Autodesk Inventor part; units mm, degrees
ref_plane "YZ Plane" through (0, 0, 0) normal (1, 0, 0) x (0, 1, 0)
ref_plane "XZ Plane" through (0, 0, 0) normal (0, 1, 0) x (-1, 0, 0)
ref_plane "XY Plane" through (0, 0, 0) normal (0, 0, 1) x (1, 0, 0)
sketch "Sketch1" plane through (0, 0, 0) normal (0, 0, 1) x (1, 0, 0)
  line L0 (-20, -20) -> (20, -20)
  line L1 (20, -20) -> (20, 20)
  line L2 (20, 20) -> (-20, 20)
  line L3 (-20, 20) -> (-20, -20)
  line L4 (-20, -20) -> (20, 20) construction
  line L5 (20, -20) -> (-20, 20) construction
  point P0 (0, 0)
  dimension "d0" = 40
  dimension "d1" = 40
extrude "Extrusion1" add sketch "Sketch1" along normal blind 5
sketch "Sketch2" plane through (0, 0, 5) normal (0, 0, 1) x (1, 0, 0)
  line L0 (-10, -10) -> (10, -10)
  line L1 (10, -10) -> (10, 10)
  line L2 (10, 10) -> (-10, 10)
  line L3 (-10, 10) -> (-10, -10)
  line L4 (-10, -10) -> (10, 10) construction
  line L5 (10, -10) -> (-10, 10) construction
  point P0 (0, 0)
  dimension "d4" = 20
  dimension "d5" = 20
extrude "Extrusion2" add sketch "Sketch2" along normal blind 5
sketch "Sketch3" plane through (0, 0, 0) normal (0, 0, -1) x (-1, 0, 0)
  line L0 (-20, -20) -> (20, -20)
  line L1 (20, -20) -> (20, 20)
  line L2 (20, 20) -> (-20, 20)
  line L3 (-20, 20) -> (-20, -20)
  line L4 (-20, -20) -> (20, 20) construction
  line L5 (20, -20) -> (-20, 20) construction
  line L6 (-10.1, -10) -> (10.1, -10)
  line L7 (10.1, -10) -> (10.1, 20)
  line L8 (10.1, 20) -> (-10.1, 20)
  line L9 (-10.1, 20) -> (-10.1, -10)
  line L10 (-10.1, -10) -> (10.1, 20) construction
  line L11 (10.1, -10) -> (-10.1, 20) construction
  point P0 (0, 0)
  point P1 (0, 5)
  dimension "d8" = 40
  dimension "d9" = 40
  dimension "d10" = 20.2
  dimension "d11" = 30
  dimension "d55" = 20
extrude "Extrusion3" add sketch "Sketch3" along normal blind 40.1 contours L3 L2 L9 L6 L7 L1 L0
sketch "Sketch4" plane through (0, 0, 0) normal (0, 0, -1) x (-1, 0, 0)
  circle A0 centre (0, 0) radius 7.5
  dimension "d14" = 15
extrude "Extrusion4" cut sketch "Sketch4" against normal blind 6
sketch "Sketch6" plane through (20, -20, -40.1) normal (1, 0, 0) x (0, 0, -1)
  line L0 (-45.1, 40) -> (-37.1, 40)
  line L1 (-37.1, 40) -> (-37.1, 0)
  line L2 (-37.1, 0) -> (-45.1, 0)
  line L3 (-45.1, 0) -> (-45.1, 40)
  line L4 (-45.1, 40) -> (-37.1, 0) construction
  line L5 (-37.1, 40) -> (-45.1, 0) construction
  line L6 (0, 40) -> (-45.1, 40)
  line L7 (-45.1, 0) -> (0, 0)
  line L8 (-45.1, 0) -> (-45.1, 40)
  point P0 (-40.1, 20)
  point P1 (-41.1, 20)
  point P2 (-40.1, 40)
  point P3 (-45.1, 50)
  dimension "d19" = 8
extrude "Extrusion6" add sketch "Sketch6" along normal blind 15
mirror "Mirror1" about plane through (0, 0, 0) normal (1, 0, 0) of "Extrusion6"
sketch "Sketch7" plane through (0, 0, 5) normal (0, 0, 1) x (1, 0, 0)
  circle A0 centre (27.5, 10) radius 2.05
  circle A1 centre (27.5, -10) radius 2.05
  circle A2 centre (-27.5, -10) radius 2.05
  circle A3 centre (-27.5, 10) radius 2.05
  line L0 (35, 20) -> (35, -20)
  line L1 (-35, 20) -> (-35, -20)
  line L2 (35, -20) -> (-35, -20)
  line L3 (-35, 20) -> (35, 20)
  line L4 (-20, 20) -> (-35, 20)
  point P0 (0, 0)
  point P1 (20, 20)
  dimension "d22" = 4.1
  dimension "d23" = 4.1
  dimension "d24" = 4.1
  dimension "d25" = 4.1
  dimension "d26" = 7.5
  dimension "d27" = 7.5
  dimension "d28" = 7.5
  dimension "d29" = 7.5
  dimension "d30" = 10
  dimension "d31" = 10
  dimension "d32" = 10
  dimension "d33" = 10
extrude "Extrusion7" cut sketch "Sketch7" against normal through all contours A0 | A1 | A2 | A3
sketch "Sketch9" plane through (20, -20, -3) normal (0, 0, -1) x (-1, 0, 0)
  circle A0 centre (-7.5, 30) radius 2.05
  circle A1 centre (-7.5, 10) radius 2.05
  circle A2 centre (47.5, 30) radius 2.05
  circle A3 centre (47.5, 10) radius 2.05
  circle A4 centre (-7.5, 30) radius 5
  circle A5 centre (-7.5, 10) radius 5
  circle A6 centre (47.5, 30) radius 5
  circle A7 centre (47.5, 10) radius 5
  point P0 (20, 20)
  dimension "d39" = 10
  dimension "d40" = 10
  dimension "d41" = 10
  dimension "d42" = 10
extrude "Extrusion8" cut sketch "Sketch9" against normal blind 5 contours A0 | A1 | A4 | A5 | A6 | A7
sketch "Sketch10" plane through (-20, -20, -40.1) normal (-1, 0, 0) x (0, 0, 1)
  line L0 (22.1, 17.5) -> (37.1, 17.5)
  line L1 (37.1, 17.5) -> (37.1, 32.5)
  line L2 (37.1, 32.5) -> (22.1, 32.5)
  line L3 (22.1, 32.5) -> (22.1, 17.5)
  line L4 (22.1, 17.5) -> (37.1, 32.5) construction
  line L5 (37.1, 17.5) -> (22.1, 32.5) construction
  line L6 (37.1, 0) -> (37.1, 40)
  line L7 (40.1, 10) -> (0, 10)
  point P0 (40.1, 20)
  point P1 (29.6, 25)
  dimension "d45" = 15
  dimension "d46" = 15
  dimension "d47" = 7.5
extrude "Extrusion9" cut sketch "Sketch10" against normal through all
sketch "Sketch11" plane through (-20, -20, -40.1) normal (0, -1, 0) x (1, 0, 0)
  line L0 (27.5, 22.1) -> (12.5, 22.1)
  line L1 (12.5, 22.1) -> (12.5, 37.1)
  line L2 (12.5, 37.1) -> (27.5, 37.1)
  line L3 (27.5, 37.1) -> (27.5, 22.1)
  line L4 (27.5, 22.1) -> (12.5, 37.1) construction
  line L5 (12.5, 22.1) -> (27.5, 37.1) construction
  line L6 (0, 37.1) -> (-15, 37.1)
  line L7 (0, 0) -> (0, 37.1)
  point P0 (20, 40.1)
  point P1 (20, 29.6)
  dimension "d50" = 15
  dimension "d51" = 15
  dimension "d52" = 20
extrude "Extrusion10" cut sketch "Sketch11" against normal through all
sketch "Sketch12" plane through (0, 0, 0) normal (0, 0, -1) x (-1, 0, 0)
  ellipse E0 centre (7.952, -7.882) end of major axis (8.818, -8.748) minor radius 1 (8.1756, -9) -> (9.07, -8.1056) ccw
  line L0 (-8.1756, -9) -> (8.1756, -9)
  ellipse E1 centre (-7.952, -7.882) end of major axis (-8.818, -8.748) minor radius 1 (-9.07, -8.1056) -> (-8.1756, -9) ccw
  line L1 (-9.07, 28.2056) -> (-9.07, -8.1056)
  ellipse E2 centre (-7.952, 27.982) end of major axis (-8.818, 28.848) minor radius 1 (-8.1756, 29.1) -> (-9.07, 28.2056) ccw
  line L2 (8.1756, 29.1) -> (-8.1756, 29.1)
  ellipse E3 centre (7.952, 27.982) end of major axis (8.818, 28.848) minor radius 1 (9.07, 28.2056) -> (8.1756, 29.1) ccw
  line L3 (9.07, -8.1056) -> (9.07, 28.2056)
  circle A0 centre (-7.525, 27.6) radius 0.7835
  circle A1 centre (7.525, 27.6) radius 0.7835
  circle A2 centre (-7.525, 12.5) radius 0.7835
  circle A3 centre (7.525, 12.5) radius 0.7835
  circle A4 centre (-7.525, -7.5) radius 0.7835
  circle A5 centre (7.525, -7.5) radius 0.7835
  circle A6 centre (0, 0) radius 6.4
  point P0 (0, 0)
hole "Hole1" at (-7.525, -7.5, 0) at (-7.525, 12.5, 0) at (7.525, 12.5, 0) at (7.525, -7.5, 0) direction (0, 0, 1) diameter 2.1 end through all
sketch "Sketch13" plane through (0, 0, 5) normal (0, 0, 1) x (1, 0, 0)
  circle A0 centre (-7.525, 12.5) radius 1.05
  circle A1 centre (7.525, 12.5) radius 1.05
  circle A2 centre (-7.525, 12.5) radius 2
  circle A3 centre (7.525, 12.5) radius 2
  point P0 (0, 0)
  dimension "d63" = 4
  dimension "d64" = 4
sketch "Sketch14" plane through (0, 0, 10) normal (0, 0, 1) x (1, 0, 0)
  circle A0 centre (-7.525, -7.5) radius 1.05
  circle A1 centre (7.525, -7.5) radius 1.05
  circle A2 centre (-7.525, -7.5) radius 2
  circle A3 centre (7.525, -7.5) radius 2
  point P0 (0, 0)
  dimension "d65" = 4
  dimension "d66" = 4
extrude "Extrusion11" cut sketch "Sketch13" against normal blind 2.5 contours A0 | A1 | A2 | A3
extrude "Extrusion12" cut sketch "Sketch14" against normal blind 2.5 contours A0 | A1 | A2 | A3
sketch "Sketch15" plane through (20, -20, -40.1) normal (1, 0, 0) x (0, 0, -1)
  line L0 (-10, 0) -> (0, 0)
  line L1 (0, 0) -> (0, 40)
  line L2 (0, 40) -> (-10, 40)
  line L3 (-10, 40) -> (-10, 0)
  line L4 (-10, 0) -> (0, 40) construction
  line L5 (0, 0) -> (-10, 40) construction
  line L6 (0, 40) -> (0, 0)
  line L7 (0, 40) -> (-37.1, 40)
  line L8 (-37.1, 0) -> (0, 0)
  point P0 (-40.1, 20)
  point P1 (-5, 20)
  dimension "d71" = 10
extrude "Extrusion13" add sketch "Sketch15" along normal blind 25
mirror "Mirror2" about plane through (0, 0, 0) normal (1, 0, 0) of "Extrusion13"
sketch "Sketch16" plane through (0, 0, -40.1) normal (0, 0, -1) x (-1, 0, 0)
  circle A0 centre (37.5, 12.5) radius 2.05
  line L0 (45, -20) -> (45, 20)
  line L1 (10.1, 20) -> (45, 20)
  circle A1 centre (37.5, -12.5) radius 2.05
  circle A2 centre (-37.5, 12.5) radius 2.05
  circle A3 centre (-37.5, -12.5) radius 2.05
  line L2 (45, -20) -> (-45, -20)
  line L3 (-45, -20) -> (-45, 20)
  line L4 (-10.1, 20) -> (-45, 20)
  point P0 (0, 0)
  dimension "d74" = 4.1
  dimension "d75" = 7.5
  dimension "d76" = 7.5
  dimension "d77" = 4.1
  dimension "d78" = 4.1
  dimension "d79" = 4.1
  dimension "d80" = 7.5
  dimension "d81" = 7.5
  dimension "d82" = 7.5
  dimension "d83" = 7.5
  dimension "d84" = 7.5
  dimension "d85" = 7.5
extrude "Extrusion14" cut sketch "Sketch16" against normal through all
sketch "Sketch17" plane through (20, -20, -30.1) normal (0, 0, 1) x (1, 0, 0)
  circle A0 centre (17.5, 7.5) radius 2.05
  circle A1 centre (17.5, 32.5) radius 2.05
  circle A2 centre (-57.5, 7.5) radius 2.05
  circle A3 centre (-57.5, 32.5) radius 2.05
  circle A4 centre (17.5, 32.5) radius 5
  circle A5 centre (17.5, 7.5) radius 5
  circle A6 centre (-57.5, 32.5) radius 5
  circle A7 centre (-57.5, 7.5) radius 5
  point P0 (-20, 20)
  dimension "d88" = 10
  dimension "d89" = 10
  dimension "d90" = 10
  dimension "d91" = 10
extrude "Extrusion15" cut sketch "Sketch17" against normal blind 5
ref_plane "Work Plane1" through (0, 0, 0) normal (1, 0, 0) x (0, 1, 0)
properties part number "motor1_bracket" material "ABS Plastic"
For this review, take the finished solid that the model builds, in its own axes (mm). A direction names the side the tool comes from. Coordinates: 2 decimals unless noted, no trailing zeros. Order: outer loops, then holes, each group sorted by start corner. A loop starts at its lowest first (then second) coordinate and runs counter-clockwise, first axis right, second up. Notation, with made-up numbers: (26, 24.5) - (84, 24.5) arc R23 ccw to (84, 43.5) - close; hole circle Ø5 at (60, 45). An arc over 180 degrees is marked (long way). Answer as a JSON object with one key per item and string values. Group by question number.
1. We need section C-C on y = 0. State the section outline as (x, z) points.
2. For faces 1 (the flat face through (-15, 5, -18)), 2 (the flat face through (27.6, 7.8, 2)), 3 (the flat face through (0, 9, 0)), 4 (the flat face through (1, -20, -23)), 5 (the cylindrical face through (7.265, -5.517, 8.768)), list the 3-axis set-ups (+Z, -Z, +X, -X, +Y, -Y) from which the entire face can be reached by the end or side of a thin tool; tool diameter is ignored.
3. We need section B-B on z = -33. State the section outline as (x, y) points.
4. We need section A-A on x = 37.5. State the section outline as (y, z) points, then the cut area to 3 significant figures.
5. For probe 1 along Y at (x, z) = (27.5, 0.55); probe 2 along X at (y, z) = (13, -10); probe 3 along Y at (x, z) = (27.5, 3.05), list the stretches that pass through material, from the lowest coordinate up.
6. Clearance check with flat-ended pins moving along their axes: P1, Ø1.5, axis at y = 4, z = 7.5, coming from the +X side; P2, Ø11, axis at x = 36, y = 15, coming from the +Z side; P3, Ø3.5, axis at x = 7.525, y = 12.5, coming from the -Z side; P4, Ø2.5, axis at x = 37.5, y = -12.5, coming from the -Z side. State where each tip first meets the part, or that it passes through.
7. We need section D-D on z = -9. State the section outline as (x, y) points, then the cut area to 3 significant figures.
8. The part is to be moulded in two halves that separate along X. For faces 6 (the flat face through (0, 0, 10)), 7 (the flat face through (0, 0, 6)), say which applies: pulls with the +X half, pulls with the -X half, needs draft (parallel to the pull), parting line crosses it, or undercut.
Final values:
{
 "1": {"outline": "(-45, -40.1) - (-10.1, -40.1) - (-10.1, -18) - (-20, -18) - (-20, -30.1) - (-45, -30.1) - close; (-35, -3) - (-10.1, -3) - (-10.1, 0) - (-7.5, 0) - (-7.5, 6) - (7.5, 6) - (7.5, 0) - (10.1, 0) - (10.1, -3) - (35, -3) - (35, 5) - (10, 5) - (10, 10) - (-10, 10) - (-10, 5) - (-35, 5) - close; (10.1, -40.1) - (45, -40.1) - (45, -30.1) - (20, -30.1) - (20, -18) - (10.1, -18) - close"},
 "2": {"face 1": "+X, -X", "face 2": "none", "face 3": "-Z, +Y", "face 4": "+Z, -Z, +X, -X, -Y", "face 5": "+Z"},
 "3": {"outline": "(-45, -20) - (45, -20) - (45, 20) - (10.1, 20) - (10.1, -10) - (-10.1, -10) - (-10.1, 20) - (-45, 20) - close; hole circle Ø10 at (-37.5, -12.5); hole circle Ø10 at (-37.5, 12.5); hole circle Ø10 at (37.5, -12.5); hole circle Ø10 at (37.5, 12.5)"},
 "4": {"outline": "(-20, -40.1) - (-14.55, -40.1) - (-14.55, -35.1) - (-17.5, -35.1) - (-17.5, -30.1) - (-20, -30.1) - close; (-10.45, -40.1) - (10.45, -40.1) - (10.45, -35.1) - (7.5, -35.1) - (7.5, -30.1) - (-7.5, -30.1) - (-7.5, -35.1) - (-10.45, -35.1) - close; (14.55, -40.1) - (20, -40.1) - (20, -30.1) - (17.5, -30.1) - (17.5, -35.1) - (14.55, -35.1) - close", "area": "259 mm²"},
 "5": {"probe 1": "-20 to -15, -5 to 5, 15 to 20", "probe 2": "-20 to -10.1, 10.1 to 20", "probe 3": "-20 to -12.05, -7.95 to 7.95, 12.05 to 20"},
 "6": {"P1": "x = 10", "P2": "z = 5", "P3": "z = 0", "P4": "through"},
 "7": {"outline": "(-20, -20) - (-7.5, -20) - (-7.5, -10) - (-10.1, -10) - (-10.1, -2.5) - (-20, -2.5) - close; (-20, 12.5) - (-10.1, 12.5) - (-10.1, 20) - (-20, 20) - close; (7.5, -20) - (20, -20) - (20, -2.5) - (10.1, -2.5) - (10.1, -10) - (7.5, -10) - close; (10.1, 12.5) - (20, 12.5) - (20, 20) - (10.1, 20) - close", "area": "547 mm²"},
 "8": {"face 6": "needs draft", "face 7": "undercut"}
}
